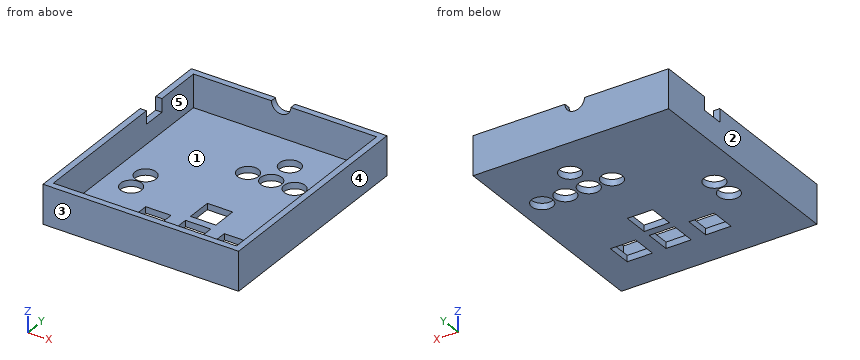
```python
from build123d import *

# Parameters (mm, degrees)
SKETCH1_W           = 50.2
SKETCH1_H           = 57.4
BOSS_EXTRUDE1_DEPTH = 10
SHELL1_T            = -1.6
SKETCH2_R           = 2.7
CUT_EXTRUDE1_DEPTH  = 10
SKETCH3_W           = 3.4
SKETCH3_H           = 6
CUT_EXTRUDE2_DEPTH  = 10
SKETCH4_R           = 2.5
CUT_EXTRUDE3_DEPTH  = 10
SKETCH5_W           = 6.5
SKETCH5_H           = 6.5
CUT_EXTRUDE4_DEPTH  = 10


with BuildPart() as part:
    # Sketch1 → Boss-Extrude1 (new body)
    with BuildSketch(Plane.XY):
        with Locations((25.1, 24.846666667)):
            Rectangle(SKETCH1_W, SKETCH1_H)
    extrude(amount=BOSS_EXTRUDE1_DEPTH)

    # Shell1
    shell1_openings = [part.faces().sort_by_distance(p)[0] for p in [
        (25.1, 24.846666667, 10),
    ]]
    offset(amount=SHELL1_T, openings=shell1_openings, kind=Kind.INTERSECTION)

    # Sketch2 → Cut-Extrude1 (cut)
    with BuildSketch(Plane(origin=(0, 0, 0), x_dir=(-1, 0, 0), z_dir=(0, 0, -1))):
        with Locations((-8.55, 17.346666667)):
            Circle(SKETCH2_R)
        with Locations((-8.55, 22.946666667)):
            Circle(SKETCH2_R)
        with Locations((-44.15, 35.896666667)):
            Circle(SKETCH2_R)
        with Locations((-26.25, 35.896666667)):
            Circle(SKETCH2_R)
        with Locations((-38.2, 35.896666667)):
            Circle(SKETCH2_R)
        with Locations((-32.2, 35.896666667)):
            Circle(SKETCH2_R)
        with Locations((-32.2, 43.096666667)):
            Circle(SKETCH2_R)
    extrude(amount=-CUT_EXTRUDE1_DEPTH, mode=Mode.SUBTRACT)

    # Sketch3 → Cut-Extrude2 (cut)
    with BuildSketch(Plane.ZY):
        with Locations((8.3, 36.746666667)):
            Rectangle(SKETCH3_W, SKETCH3_H)
    extrude(amount=-CUT_EXTRUDE2_DEPTH, mode=Mode.SUBTRACT)

    # Sketch4 → Cut-Extrude3 (cut)
    with BuildSketch(Plane(origin=(0, 53.546666667, 0), x_dir=(1, 0, 0), z_dir=(0, 1, 0))):
        with Locations((24.1, -10)):
            Circle(SKETCH4_R)
    extrude(amount=-CUT_EXTRUDE3_DEPTH, mode=Mode.SUBTRACT)

    # Sketch5 → Cut-Extrude4 (cut)
    with BuildSketch(Plane(origin=(0, 0, 0), x_dir=(-1, 0, 0), z_dir=(0, 0, -1))):
        with Locations((-39.15, 8.896666667)):
            Rectangle(SKETCH5_W, SKETCH5_H)
        with Locations((-29.2, 8.896666667)):
            Rectangle(SKETCH5_W, SKETCH5_H)
        with Locations((-19, 8.896666667)):
            Rectangle(SKETCH5_W, SKETCH5_H)
        with Locations((-29.2, 17.346666667)):
            Rectangle(SKETCH5_W, SKETCH5_H)
    extrude(amount=-CUT_EXTRUDE4_DEPTH, mode=Mode.SUBTRACT)


solid = part.part
```
The listing builds one solid part. Answer for the finished solid, in the listing's coordinates (mm). Face numbers are marked on the shaded views. A direction names the side the tool comes from. Round coordinates to 2 decimals unless told otherwise and drop trailing zeros. Write each loop counter-clockwise with the first axis right and the second up, starting at its lowest first coordinate (ties: lowest second). Pieces come first, ordered by that corner, then holes. Notation, with made-up numbers: (-21, 42) -> (5, 42) arc R21 cw to (5, 68) -> close; hole circle Ø11 at (75.5, 35). An arc over 180 degrees is marked (long way). Answer as a JSON object with one key per item and string values. Group by question number.
Q1. Section B-B (y = 7) is taken. Write down the section's boundary in (x, z).
Q2. Section A-A (x = 8.55) is taken. Write down the section's boundary in (y, z).
Q3. This flat-tipped pin is pushed along its axis until it touches: pin 1 Ø14 at (x, y) = (28.5, 38) entering from +Z. Where does it stop, or does it pass through?
Q4. Section D-D (x = 16.5) is taken. Write down the section's boundary in (y, z).
Q5. Which of the six approach directions +Z, -Z, +X, -X, +Y, -Y give full straight-line access (tool end or side, diameter ignored) to the marked faces 1 and 2?
Q6. Section C-C (z = 5.5) is taken. Write down the section's boundary in (x, y), plus the area to 3 significant figures.
Q7. Determine the mould class of the marked faces 3, 4 and 5 for opening direction X: pulls with the +X half, pulls with the -X half, needs draft (parallel to the pull), parting line crosses it, or undercut.
Q8. Straight lines are drawn through the part: line 1 along Y through (x, z) = (32.2, 1.25); line 2 along Y through (x, z) = (26.25, 1.05); line 3 along Y through (x, z) = (38.2, 0.9). For each, find the intervals that lie inside material, in ascending order.
Check values:
{
 "1": {"outline": "(0, 0) -> (15.75, 0) -> (15.75, 1.6) -> (1.6, 1.6) -> (1.6, 10) -> (0, 10) -> close; (22.25, 0) -> (25.95, 0) -> (25.95, 1.6) -> (22.25, 1.6) -> close; (32.45, 0) -> (35.9, 0) -> (35.9, 1.6) -> (32.45, 1.6) -> close; (42.4, 0) -> (50.2, 0) -> (50.2, 10) -> (48.6, 10) -> (48.6, 1.6) -> (42.4, 1.6) -> close"},
 "2": {"outline": "(-3.85, 0) -> (14.65, 0) -> (14.65, 1.6) -> (-2.25, 1.6) -> (-2.25, 10) -> (-3.85, 10) -> close; (20.05, 0) -> (20.25, 0) -> (20.25, 1.6) -> (20.05, 1.6) -> close; (25.65, 0) -> (53.55, 0) -> (53.55, 10) -> (51.95, 10) -> (51.95, 1.6) -> (25.65, 1.6) -> close"},
 "3": {"pin 1": "z = 1.6"},
 "4": {"outline": "(-3.85, 0) -> (5.65, 0) -> (5.65, 1.6) -> (-2.25, 1.6) -> (-2.25, 10) -> (-3.85, 10) -> close; (12.15, 0) -> (53.55, 0) -> (53.55, 10) -> (51.95, 10) -> (51.95, 1.6) -> (12.15, 1.6) -> close"},
 "5": {"face 1": "+Z", "face 2": "+Z, -Z, -X, +Y, -Y"},
 "6": {"outline": "(0, -3.85) -> (50.2, -3.85) -> (50.2, 53.55) -> (0, 53.55) -> close; hole (1.6, -2.25) -> (48.6, -2.25) -> (48.6, 51.95) -> (1.6, 51.95) -> close", "area": "334 mm^2"},
 "7": {"face 3": "needs draft", "face 4": "pulls with the +X half", "face 5": "undercut"},
 "8": {"line 1": "-3.85 to 5.65, 12.15 to 14.1, 20.6 to 33.2, 38.6 to 40.4, 45.8 to 53.55", "line 2": "-3.85 to 5.65, 12.15 to 14.1, 20.6 to 33.2, 38.6 to 53.55", "line 3": "-3.85 to 5.65, 12.15 to 33.2, 38.6 to 53.55"}
}
